Verification items for the finished model (mm, model axes). A direction names the side the tool comes from. Round coordinates to 2 decimals unless told otherwise and drop trailing zeros. Write each loop counter-clockwise with the first axis right and the second up, starting at its lowest first coordinate (ties: lowest second). Pieces come first, ordered by that corner, then holes.
from build123d import *

# Parameters (mm, degrees)
F0_W     = 32
F0_H     = 32
F1_DEPTH = 3
F2_W     = 32
F2_H     = 10
F3_DEPTH = 50
F5_DEPTH = 30
F6_F1_R  = 1
F6_F2_R  = 1


with BuildPart() as f1:
    # F0 (on Top) → F1 (new body)
    with BuildSketch(Plane.XY):
        Rectangle(F0_W, F0_H)
    extrude(amount=F1_DEPTH)

    # F2 (on face) → F3 (join)
    with BuildSketch(Plane.XY.offset(3)):
        Rectangle(F2_W, F2_H)
    extrude(amount=F3_DEPTH)

    # F4 (on face) → F5 (cut)
    with BuildSketch(Plane.XY.offset(53)):
        Polygon((10.8576942235, 5), (-10.8576942235, 5), (-10.8576942235, 2), (-13.5, 2), (-13.5, -2), (-10.8576942235, -2), (-10.8576942235, -5), (10.8576942235, -5), (10.8576942235, -2), (13.5, -2), (13.5, 2), (10.8576942235, 2), align=None)
    extrude(amount=-F5_DEPTH, mode=Mode.SUBTRACT)

    # F6: fillet of radius 1 on 32 edges, made by hand

    # F6_f1
    f6_f1_edges = [f1.edges().sort_by_distance(p)[0] for p in [
        (0, -5, 3),
        (0, 5, 3),
    ]]
    fillet(f6_f1_edges, radius=F6_F1_R)

    # F6_f2
    f6_f2_edges = [f1.edges().sort_by_distance(p)[0] for p in [
        (0, 16, 0),
        (-16, 0, 0),
        (0, -16, 0),
        (16, 0, 0),
        (16, -5, 28.5),
        (13.4288471118, -5, 53),
        (10.8576942235, -5, 38),
        (0, -5, 23),
        (-10.8576942235, -5, 38),
        (-13.4288471118, -5, 53),
        (-16, -5, 28.5),
        (-16, 5, 28.5),
        (-13.4288471118, 5, 53),
        (-10.8576942235, 5, 38),
        (0, 5, 23),
        (10.8576942235, 5, 38),
        (13.4288471118, 5, 53),
        (16, 5, 28.5),
        (16, 0, 53),
        (10.8576942235, -3.5, 53),
        (12.1788471118, -2, 53),
        (13.5, 0, 53),
        (12.1788471118, 2, 53),
        (10.8576942235, 3.5, 53),
        (-10.8576942235, 3.5, 53),
        (-12.1788471118, 2, 53),
        (-13.5, 0, 53),
        (-12.1788471118, -2, 53),
        (-10.8576942235, -3.5, 53),
        (-16, 0, 53),
        (16, 5.2928932188, 3.2928932188),
        (-16, 5.2928932188, 3.2928932188),
        (-16, -5.2928932188, 3.2928932188),
        (16, -5.2928932188, 3.2928932188),
    ]]
    fillet(f6_f2_edges, radius=F6_F2_R)


solid = f1.part
Q1. Sectioned sample at D-D (z = 8). Enter the section's corners in (x, y), plus the area to 3 significant figures.
Recorded:
outline: (-16, -4) arc R1 ccw to (-15, -5) - (15, -5) arc R1 ccw to (16, -4) - (16, 4) arc R1 ccw to (15, 5) - (-15, 5) arc R1 ccw to (-16, 4) - close
area: 319 mm2
Q2. Release check for a two-part mould opening along Y. For faces 1 (the flat face through (16, 0, 24)), 2 (the flat face through (0, 16, 2)), 3 (the flat face through (12, 2, 38)) record: released by +Y, released by -Y, zero draft, split by the parting line, or undercut.
Recorded:
face 1: zero draft
face 2: released by +Y
face 3: undercut
Q3. Material ranges on line 1 along X through (y, z) = (1, 32); line 2 along Y through (x, z) = (-14, 21); line 3 along Z through (x, y) = (8, 8.5), recorded low to high.
Recorded:
line 1: x = -16 to -13.5, 13.5 to 16
line 2: y = -5 to 5
line 3: z = 0 to 3
Q4. Sectioned sample at B-B (x = 3.5). Enter the section's corners in (y, z).
Recorded:
outline: (-16, 1) arc R1 ccw to (-15, 0) - (15, 0) arc R1 ccw to (16, 1) - (16, 3) - (6, 3) arc R1 cw to (5, 4) - (5, 22) arc R1 ccw to (4, 23) - (-4, 23) arc R1 ccw to (-5, 22) - (-5, 4) arc R1 cw to (-6, 3) - (-16, 3) - close
Q5. Sectioned sample at A-A (z = 36.5). Enter the section's corners in (x, y).
Recorded:
outline: (-16, -4) arc R1 ccw to (-15, -5) - (-11.86, -5) arc R1 ccw to (-10.86, -4) - (-10.86, -2) - (-13.5, -2) - (-13.5, 2) - (-10.86, 2) - (-10.86, 4) arc R1 ccw to (-11.86, 5) - (-15, 5) arc R1 ccw to (-16, 4) - close; (10.86, -4) arc R1 ccw to (11.86, -5) - (15, -5) arc R1 ccw to (16, -4) - (16, 4) arc R1 ccw to (15, 5) - (11.86, 5) arc R1 ccw to (10.86, 4) - (10.86, 2) - (13.5, 2) - (13.5, -2) - (10.86, -2) - close
Q6. Tool access check on faces 4 (the flat face through (0, -5, 17)), 5 (the flat face through (0, 11, 3)), 6 (the flat face through (13.5, 0, 38)), 7 (the flat face through (-10.858, 3, 38)). Record the directions out of +Z, -Z, +X, -X, +Y, -Y that give a thin tool (end or side, any length) a straight path to the whole face; none if there is none.
Recorded:
face 4: +Z, +X, -X, -Y
face 5: +Z, +X, -X, +Y
face 6: +Z
face 7: +Z, +Y, -Y
Q7. Depth check by flat-ended pin: P1, Ø2, axis at x = 12.5, z = 37, coming from the +Y side; P2, Ø5, axis at x = 2, y = -10.5, coming from the +Z side; P3, Ø6, axis at x = 12.5, z = 10.5, coming from the -Y side. Enter the tip coordinate at first touch or a pass-through.
Recorded:
P1: stops at y = 5
P2: stops at z = 3
P3: stops at y = -5
Q8. Sectioned sample at C-C (y = -12). Enter the section's corners in (x, z).
Recorded:
outline: (-16, 1) arc R1 ccw to (-15, 0) - (15, 0) arc R1 ccw to (16, 1) - (16, 2) arc R1 ccw to (15, 3) - (-15, 3) arc R1 ccw to (-16, 2) - close
